from build123d import *

# Parameters (mm, degrees)
CROQUIS2_R              = 1.95
SALIENTE_EXTRUIR1_DEPTH = 8
C_PULA1_FACE_RADIUS     = 1.95
C_PULA1_HEIGHT          = 5.3
CROQUIS15_R             = 20
SALIENTE_EXTRUIR2_DEPTH = 2
FILLET1_R               = 2
SKETCH1_R               = 19
CUT_EXTRUDE1_DEPTH      = 0.5


with BuildPart() as part:
    # Croquis2 → Saliente-Extruir1 (new body)
    with BuildSketch(Plane(origin=(0, 0, 0), x_dir=(1, 0, 0), z_dir=(0, 1, 0))):
        with Locations(Location((0, 0, 0), (0, 0, 270))):
            Circle(CROQUIS2_R)
    extrude(amount=SALIENTE_EXTRUIR1_DEPTH)

    # Cúpula1: a dome of height H over a round flat face of radius A is a cap of a sphere of radius (A * A + H * H) / (2 * H)
    c_pula1_r = (C_PULA1_FACE_RADIUS * C_PULA1_FACE_RADIUS + C_PULA1_HEIGHT * C_PULA1_HEIGHT) / (2 * C_PULA1_HEIGHT)
    c_pula1_base = Plane((0, 8, 0), z_dir=(0, 1, 0))
    with Locations(c_pula1_base.offset(C_PULA1_HEIGHT - c_pula1_r)):
        c_pula1_ball = Sphere(c_pula1_r, mode=Mode.PRIVATE)
    add(split(c_pula1_ball, bisect_by=c_pula1_base, keep=Keep.TOP, mode=Mode.PRIVATE))

    # Croquis15 → Saliente-Extruir2 (add)
    with BuildSketch(Plane(origin=(0, 0, 0), x_dir=(-1, 0, 0), z_dir=(0, -1, 0))):
        with Locations(Location((0, 0, 0), (0, 0, 90))):
            Circle(CROQUIS15_R)
    extrude(amount=SALIENTE_EXTRUIR2_DEPTH)

    # Fillet1
    fillet1_edges = [part.edges().sort_by_distance(p)[0] for p in [
        (0, 8, -1.95),
        (0, 0, -1.95),
    ]]
    fillet(fillet1_edges, radius=FILLET1_R)

    # Sketch1 → Cut-Extrude1 (cut)
    with BuildSketch(Plane.XZ.offset(2)):
        with Locations(Location((0, 0, 0), (0, 0, 270))):
            Circle(SKETCH1_R)
    extrude(amount=-CUT_EXTRUDE1_DEPTH, mode=Mode.SUBTRACT)


solid = part.part
The model under review builds one solid part; all positions refer to its coordinate system, in mm. A direction names the side the tool comes from. Give positions to 0.01 mm unless a question says otherwise; leave off trailing zeros. Order: outer loops, then holes, each group sorted by start corner. A loop starts at its lowest first (then second) coordinate and runs counter-clockwise, first axis right, second up. Notation, with made-up numbers: M -35,84.25 L 2,84.25 A24 ccw 2,99.25 Z; hole C -24.75,67 d3. An arc over 180 degrees is marked long. Use one line per item in the form item = value. Start each with the question number.
Item 1: For faces 1 (the flat face through (0, -1.5, 0)), 2 (the cylindrical face through (-19.524, -0.986, 4.336)), list the 3-axis set-ups (+Z, -Z, +X, -X, +Y, -Y) from which the entire face can be reached by the end or side of a thin tool; tool diameter is ignored.
Item 2: We need section A-A on x = 6. Give the boundary of the cut face in (y, z).
Item 3: We need section C-C on y = 10.25. Give the boundary of the cut face in (x, z), plus the area to 3 significant figures.
Item 4: To check wall thickness, follow line 1 along X through (y, z) = (-1.75, 0); line 2 along Y through (x, z) = (18.5, 5); line 3 along Y through (x, z) = (1, 6). State the ranges of each line that lie inside material, in increasing order. Write a range as from..to.
Item 5: We need section D-D on y = 5.25. Give the boundary of the cut face in (x, z), plus the area to 3 significant figures.
Item 6: The part is to be moulded in two halves that separate along Y. For faces 3 (the cylindrical face through (-11.56, -1.75, 15.08)), 4 (the flat face through (-7, -2, -18)), 5 (the cylindrical face through (-0.75, 4.57, 1.8)), 6 (the flat face through (0.3, 0, -4.2)), say which applies: pulls with the +Y half, pulls with the -Y half, needs draft (parallel to the pull), parting line crosses it, or undercut.
Item 7: Insertion check: pin 1 Ø8 at (x, y) = (5.5, 3.5) entering from +Z; pin 2 Ø6 at (x, z) = (11.5, -2.5) entering from -Y; pin 3 Ø5 at (x, y) = (-10, 0.5) entering from +Z. Each pin has a flat end and moves straight along its axis. Give the tip position at first contact, or say it passes through.
Item 8: We need section B-B on z = 8. Give the boundary of the cut face in (x, y).
Completed:
q1.face_1 = -Y
q1.face_2 = +Y, -Y
q2.outline = M -2,-19.08 L 0,-19.08 L 0,19.08 L -2,19.08 L -2,18.03 L -1.5,18.03 L -1.5,-18.03 L -2,-18.03 Z
q3.outline = C 0,0 d6.02
q3.area = 28.4 mm²
q4.line_1 = -20..-19, 19..20
q4.line_2 = -2..0
q4.line_3 = -1.5..0
q5.outline = C 0,0 d3.9
q5.area = 11.9 mm²
q6.face_3 = needs draft
q6.face_4 = pulls with the -Y half
q6.face_5 = undercut
q6.face_6 = pulls with the +Y half
q7.pin_1 = 19.68
q7.pin_2 = -1.5
q7.pin_3 = 18.52
q8.outline = M -18.33,-2 L -17.23,-2 L -17.23,-1.5 L 17.23,-1.5 L 17.23,-2 L 18.33,-2 L 18.33,0 L -18.33,0 Z
